Verification items for this drawing (mm, ordinates from the low corner). Coordinates: 2 decimals unless noted, no trailing zeros. Write each loop counter-clockwise with the first axis right and the second up, starting at its lowest first coordinate (ties: lowest second). Pieces come first, ordered by that corner, then holes. Notation, with made-up numbers: M 49,3.25 L 82,3.25 A8 ccw 82,11.25 Z; hole C 64.25,-9 d1. An arc over 180 degrees is marked long. Put each result on its own line as item: value. Start each with the question number.
1) Scan lines: line 1 along Y through (x, z) = (138, 2.8); line 2 along X through (y, z) = (136.5, 3.5); line 3 along Y through (x, z) = (137, 2.35). Record each from-to range of solid material in increasing order.
2) Gauge pin test, flat ends, axial feed: pin 1 (1 mm diameter, centred on y = 232.5, z = 1, fed in from +X) (1 decimal); pin 2 (1.5 mm diameter, centred on x = 136, z = 1.5, fed in from -Y); pin 3 (23.5 mm diameter, centred on x = 18, y = 138, fed in from -Z); pin 4 (1.5 mm diameter, centred on x = 59.5, z = 2.5, fed in from +Y). Record the tip position at first contact, or that the pin passes through.
3) Cross-section at D-D on y = 106. Record the cut outline in (x, z).
4) Cross-section at C-C on z = 1.95. Count the separate pieces of the cut face and the enclosed holes in it, plus the area to 3 significant figures.
5) Cross-section at A-A on x = 138. Record the cut outline in (y, z).
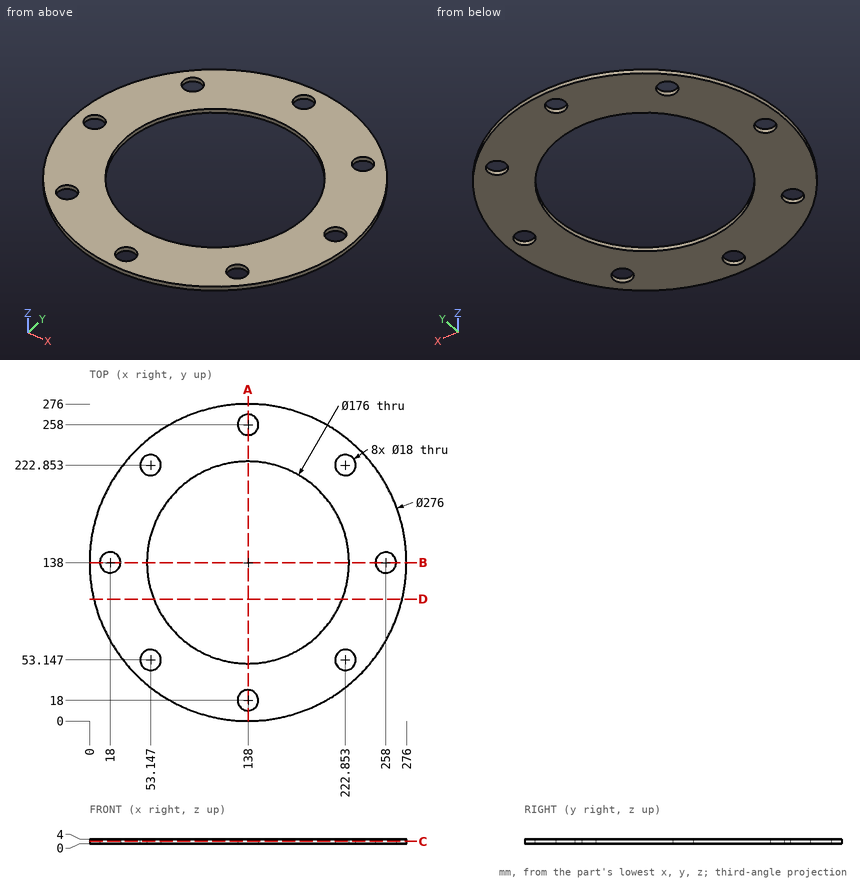
Answer key:
1. line 1: y = 0 to 9, 27 to 50, 226 to 249, 267 to 276
1. line 2: x = 0.01 to 9.13, 26.87 to 50.01, 225.99 to 249.13, 266.87 to 275.99
1. line 3: y = 0 to 9.06, 26.94 to 50.01, 225.99 to 249.06, 266.94 to 276
2. pin 1: stops at x = 239
2. pin 2: stops at y = 0.01
2. pin 3: stops at z = 0
2. pin 4: stops at y = 252.01
3. outline: M 3.76,0 L 56.02,0 L 56.02,4 L 3.76,4 Z; M 219.98,0 L 272.24,0 L 272.24,4 L 219.98,4 Z
4. separate pieces: 1
4. enclosed holes: 9
4. area: 33,500 mm²
5. outline: M 0,0 L 9,0 L 9,4 L 0,4 Z; M 27,0 L 50,0 L 50,4 L 27,4 Z; M 226,0 L 249,0 L 249,4 L 226,4 Z; M 267,0 L 276,0 L 276,4 L 267,4 Z
